from build123d import *

# Parameters (mm, degrees)
SKETCH_1_W      = 170.942557362
SKETCH_1_H      = 172.163575629
EXTRUDE_1_DEPTH = 2
SKETCH_2_W      = 50
SKETCH_2_H      = 87
EXTRUDE_2_DEPTH = 35
SKETCH_3_W      = 30.35102549
SKETCH_3_H      = 31.572043757
SKETCH_3_W_2    = 16.570962193
SKETCH_3_H_2    = 17.704764869
SKETCH_3_H_3    = 2.442036534
SKETCH_3_W_3    = 86.692296948
SKETCH_3_H_4    = 24.071502975
SKETCH_3_W_4    = 9.942577316
SKETCH_3_H_5    = 43.258932884
SKETCH_3_W_5    = 59.829895076
SKETCH_3_H_6    = 13.780063298
SKETCH_3_W_6    = 55.989922961
SKETCH_3_H_7    = 12.893447817
SKETCH_3_W_7    = 34.783578006
SKETCH_3_H_8    = 10.603172478
SKETCH_3_W_8    = 11.686889126
SKETCH_3_H_9    = 48.143005951
SKETCH_3_H_10   = 50.585042485
SKETCH_3_W_9    = 9.605807423
SKETCH_3_H_11   = 6.465349072
EXTRUDE_3_DEPTH = 14
CHAMFER_1_SIZE  = 2


with BuildPart() as part:
    # 草图1 → 凸台-拉伸1 (new body)
    with BuildSketch(Plane.XY):
        with Locations((-78.914431177, 80.434949445)):
            Rectangle(SKETCH_1_W, SKETCH_1_H)
        with BuildLine():
            ThreePointArc((-159.455, 0), (-157.48, -1.975), (-155.505, 0))
            ThreePointArc((-155.505, 0), (-157.48, 1.975), (-159.455, 0))
        make_face(mode=Mode.SUBTRACT)
        with BuildLine():
            ThreePointArc((-1.975, 0), (0, -1.975), (1.975, 0))
            ThreePointArc((1.975, 0), (0, 1.975), (-1.975, 0))
        make_face(mode=Mode.SUBTRACT)
        with BuildLine():
            ThreePointArc((-1.975, 154.919999989), (0, 152.944999989), (1.975, 154.919999989))
            ThreePointArc((1.975, 154.919999989), (0, 156.894999989), (-1.975, 154.919999989))
        make_face(mode=Mode.SUBTRACT)
        with BuildLine():
            ThreePointArc((-159.455, 132.08), (-157.48, 130.105), (-155.505, 132.08))
            ThreePointArc((-155.505, 132.08), (-157.48, 134.055), (-159.455, 132.08))
        make_face(mode=Mode.SUBTRACT)
    extrude(amount=-EXTRUDE_1_DEPTH)

    # 草图2 → 凸台-拉伸2 (add)
    with BuildSketch(Plane(origin=(0, 0, -2), x_dir=(-1, 0, 0), z_dir=(0, 0, -1))):
        with Locations((50, 87.178999994)):
            Rectangle(SKETCH_2_W, SKETCH_2_H)
    extrude(amount=EXTRUDE_2_DEPTH)

    # 草图3 → 凸台-拉伸3 (add)
    with BuildSketch(Plane(origin=(0, 0, -2), x_dir=(-1, 0, 0), z_dir=(0, 0, -1))):
        with Locations((52.052029306, 148.811972389)):
            Rectangle(SKETCH_3_W, SKETCH_3_H)
        with Locations((97.491351952, 157.664354825)):
            Rectangle(SKETCH_3_W_2, SKETCH_3_H_2)
        Polygon((150.256784199, 166.516737259), (119.905758708, 166.516737259), (119.905758708, 160.251119597), (119.905758708, 153.259967505), (150.256784199, 153.259967505), align=None)
        with Locations((97.491351952, 167.737755526)):
            Rectangle(SKETCH_3_W_2, SKETCH_3_H_3)
        Polygon((119.905758708, 166.716468669), (119.905758708, 166.516737259), (150.256784199, 166.516737259), (150.256784199, 166.716468669), (150.256784199, 174.017278041), (119.905758708, 174.017278041), align=None)
        Polygon((163.445120655, 166.516737259), (150.256784199, 166.516737259), (150.256784199, 153.259967505), (150.256784199, 151.587551841), (163.445120655, 151.587551841), align=None)
        with Locations((121.039561384, 62.555753395)):
            Rectangle(SKETCH_3_W_3, SKETCH_3_H_4)
        with Locations((159.4144212, 26.797361293)):
            Rectangle(SKETCH_3_W_4, SKETCH_3_H_5)
        with Locations((114.236745326, 1.243193279)):
            Rectangle(SKETCH_3_W_5, SKETCH_3_H_6)
        with Locations((31.520690489, 0.799885539)):
            Rectangle(SKETCH_3_W_6, SKETCH_3_H_7)
        with Locations((23.374350658, 16.168791166)):
            Rectangle(SKETCH_3_W_7, SKETCH_3_H_8)
        with Locations((-0.713402941, 105.640255096)):
            Rectangle(SKETCH_3_W_8, SKETCH_3_H_9)
        with Locations((-0.713402941, 39.356406323)):
            Rectangle(SKETCH_3_W_8, SKETCH_3_H_10)
        with Locations((115.102854997, 163.483794133)):
            Rectangle(SKETCH_3_W_9, SKETCH_3_H_11)
    extrude(amount=EXTRUDE_3_DEPTH)

    # 倒角1
    chamfer_1_edges = [part.edges().sort_by_distance(p)[0] for p in [
        (-25, 87.178999994, -37),
        (-50, 43.678999994, -37),
        (-75, 87.178999994, -37),
        (-50, 130.678999994, -37),
    ]]
    chamfer(chamfer_1_edges, length=CHAMFER_1_SIZE)


solid = part.part
Can you work these out from the model? Positions are in its coordinate system, mm. A direction names the side the tool comes from. Give positions to 0.01 mm unless a question says otherwise; leave off trailing zeros. Loops run counter-clockwise (first coordinate to the right, second up) from the corner with the lowest first, then second, coordinate; pieces in that order, holes last. Notation, with made-up numbers: M 16.25,35.25 L 46.25,35.25 A33 cw 46.25,66.25 Z; hole C 4.25,-13 d9. An arc over 180 degrees is marked long. One line per item, written item: value. Start each with the question number.
1) If we section it at C-C, the plane z = -12.5: Give the number of separate pieces and of enclosed holes in the cut face, and give its area (3 significant figures).
2) I'm going to push flat-ended pins straight in: pin 1 (24.5 mm diameter, centred on x = -47.5, y = 147.5, fed in from -Z); pin 2 (7 mm diameter, centred on x = -49, z = -6.5, fed in from +Y); pin 3 (6 mm diameter, centred on y = 81, z = -7.5, fed in from -X). Where does each tip first touch, or does it pass through?
3) If we section it at B-B, the plane x = -129: Write out the boundary of the cut face in (y, z).
4) If we section it at A-A, the plane y = 144.5: Write out the boundary of the cut face in (x, z).
5) If I drill on line 1 (Y direction, x = -126.5, z = -5); line 2 (X direction, y = 62.5, z = -10.5); line 3 (Y direction, x = 0, z = -1.2) (3 decimals), over which ranges is the centre line in solid material (lowest first)? Write a range as [from, to].
6) On a 3-axis mill with a long thin cutter (end or side, diameter ignored), from which of +Z, -Z, +X, -X, +Y, -Y can I reach the whole of each face in a straight line? I mean faces 3 (the face through (-97, 168.959, -9)), 4 (the face through (-5.13, 39, -9)), 5 (the face through (-134, 170, -2)), 6 (the face through (-97, 148.812, -9)). Say none if no direction works.
7) Thinking about a two-plate mould opening in X: for faces 1 (the face through (-75, 87, -18)), 2 (the face through (-120, 50.52, -9)), which applies, +X half, -X half, draft (parallel to the pull), parting line (faces both ways), or undercut?
8) If we section it at D-D, the plane z = -24: Write out the boundary of the cut face in (x, y), and give its area (3 significant figures).
Completed:
1. separate pieces: 11
1. enclosed holes: 0
1. area: 12,100 mm^2
2. pin 1: stops at z = -16
2. pin 2: stops at y = 164.6
2. pin 3: stops at x = -75
3. outline: M -5.65,-16 L 8.13,-16 L 8.13,-2 L 50.52,-2 L 50.52,-16 L 74.59,-16 L 74.59,-2 L 153.26,-2 L 153.26,-16 L 174.02,-16 L 174.02,-2 L 166.52,-2 L 166.52,0 L -5.65,0 Z
4. outline: M -164.39,-2 L -67.23,-2 L -67.23,-16 L -36.88,-16 L -36.88,-2 L 6.56,-2 L 6.56,0 L -164.39,0 Z
5. line 1: y = [-5.65, 8.13], [50.52, 74.59], [153.26, 174.02]
5. line 2: x = [-164.39, -77.69], [-75, -25], [-5.13, 6.56]
5. line 3: y = [-5.647, -1.975], [1.975, 152.945], [156.895, 166.517]
6. face 3: +Z, -Z, +X, +Y
6. face 4: -Z, +Y
6. face 5: +Z, +X, -X, +Y
6. face 6: -Z, -X
7. face 1: undercut
7. face 2: draft
8. outline: M -75,43.68 L -25,43.68 L -25,130.68 L -75,130.68 Z
8. area: 4,350 mm^2
